Autodesk Inventor part; units mm, degrees
ref_plane "Startebene" through (0, 0, 0) normal (1, 0, 0) x (0, 1, 0)
ref_plane "XZ Plane" through (0, 0, 0) normal (0, 1, 0) x (-1, 0, 0)
ref_plane "XY Plane" through (0, 0, 0) normal (0, 0, 1) x (1, 0, 0)
sketch "Hauptskizze" plane through (0, 0, 0) normal (0, 0, 1) x (1, 0, 0)
  line L0 (0, 0) -> (55, 0)
  line L1 (0, 0) -> (0, 3)
  line L2 (40, 3) -> (40, 2.5)
  line L3 (0, 3) -> (40, 3)
  line L4 (55, 2.5) -> (55, 0)
  line L5 (40, 2.5) -> (55, 2.5)
  dimension "d3" = 6
  dimension "d14" = 5
revolve "Umdrehung1" add sketch "Hauptskizze" angle 360 about axis through (0, 0, 0) along (1, 0, 0)
chamfer "Fase4" distance 0.5 angle 45 1 edges at (0, -3, 0) measured on face at (26.6667, 2.9612, -0.4812)
chamfer "Fase5" distance 0.5 angle 45 1 edges at (55, -2.5, 0) measured on face at (50, 2.4919, -0.2012)
properties part number "Welle 5x15+6x45" material "Steel"
Part model, mm, in its own coordinate system. A direction names the side the tool comes from. Round coordinates to 2 decimals unless told otherwise and drop trailing zeros. Order: outer loops, then holes, each group sorted by start corner. A loop starts at its lowest first (then second) coordinate and runs counter-clockwise, first axis right, second up. Notation, with made-up numbers: M -9.5,20 L 14.5,20 A20 ccw 14.5,56 Z; hole C -0.5,42 d1. An arc over 180 degrees is marked long. Answer in a Markdown table with one row per item. Add a question column.
Q1. Cut at C-C on x = 12.5. Give the cut face in (y, z).
Q2. 3-axis set-ups, long thin cutter, end or side, ignore diameter. For faces 1 (the face through (0, 0, 0)), 2 (the face through (40, -2, 2)): which of +Z, -Z, +X, -X, +Y, -Y reach the whole face in a straight line?
Q3. Cut at A-A on y = 0. Give the cut face in (x, z).
Q4. Wall check: L1, parallel to Z at x = 42.5, y = -1.5; L2, parallel to Y at x = 47, z = 0.8; L3, parallel to Y at x = 38.5, z = 0.55. Give the ranges that are in metal, low to high. Write a range as from..to.
Q5. Pin check, flat tips, straight feed: pin 1 (3 mm diameter, centred on x = 10, z = -2, fed in from +Y); pin 2 (2 mm diameter, centred on x = 44.5, z = 1.5, fed in from -Y); pin 3 (3 mm diameter, centred on x = 44.5, y = 0.5, fed in from +Z). Stop position of each tip, or through.
Established:
| question | item | result |
|---|---|---|
| 1 | outline | C 0,0 d6 |
| 2 | face 1 | +Z, -Z, -X, +Y, -Y |
| 2 | face 2 | +X |
| 3 | outline | M 0,-2.5 L 0.5,-3 L 40,-3 L 40,-2.5 L 54.5,-2.5 L 55,-2 L 55,2 L 54.5,2.5 L 40,2.5 L 40,3 L 0.5,3 L 0,2.5 Z |
| 4 | L1 | z = -2..2 |
| 4 | L2 | y = -2.37..2.37 |
| 4 | L3 | y = -2.95..2.95 |
| 5 | pin 1 | stops at y = 2.96 |
| 5 | pin 2 | stops at y = -2.45 |
| 5 | pin 3 | stops at z = 2.5 |
